Drawing for the job (mm, zero at the part's lowest x, y, z). A direction names the side the tool comes from. Give positions to 0.01 mm unless a question says otherwise; leave off trailing zeros. Write each loop counter-clockwise with the first axis right and the second up, starting at its lowest first coordinate (ties: lowest second). Pieces come first, ordered by that corner, then holes. Notation, with made-up numbers: (78, 20.5) - (96, 20.5) arc R20 cw to (96, 40.5) - close; hole circle Ø8 at (-3.5, 24.25). An arc over 180 degrees is marked (long way). Write item = value, one per line. Start each with the question number.
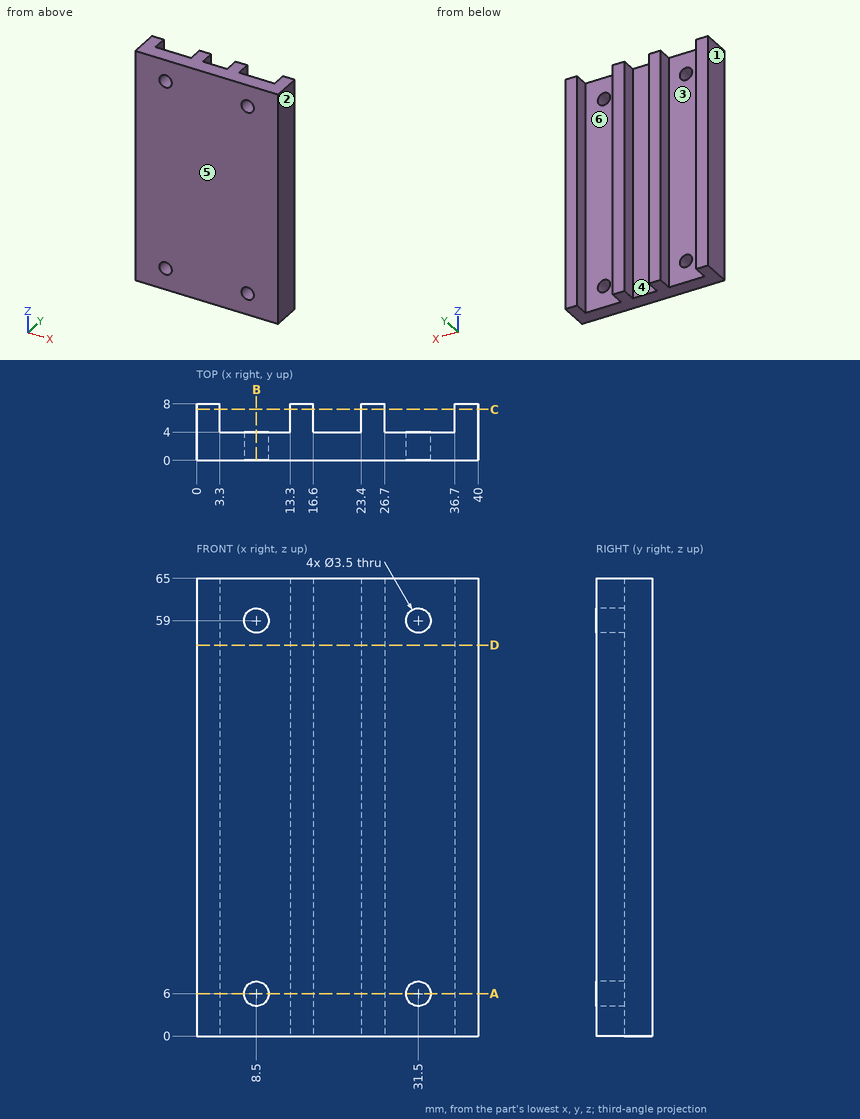
1. Pin check, flat tip, straight feed: pin 1 Ø3 at (x, z) = (6, 27) entering from +Y. Stop position of the tip, or through.
2. Wall check: line 1 along X through (y, z) = (4.25, 27); line 2 along Z through (x, y) = (31.5, 1.75); line 3 along X through (y, z) = (2.1, 6). Give the ranges that are in metal, low to high.
3. Cut at A-A (z = 6). Give the cut face in (x, y).
4. Cut at D-D (z = 55.5). Give the cut face in (x, y), then the cut area to 3 significant figures.
5. Cut at B-B (x = 8.5). Give the cut face in (y, z), then the cut area to 3 significant figures.
6. Cut at C-C (y = 7.25). Give the cut face in (x, z).
7. Mould opens along X. For the marked faces 1, 2, 3 and 4 say: +X half, -X half, draft (parallel to the pull), parting line (faces both ways), or undercut.
8. Tool access for the marked faces 5 and 6: list every direction of +Z, -Z, +X, -X, +Y, -Y with a clear straight run to the whole face (end or side of a thin tool).
Output:
q1.pin_1 = 4
q2.line_1 = 0 to 3.3, 13.3 to 16.6, 23.4 to 26.7, 36.7 to 40
q2.line_2 = 0 to 4.25, 7.75 to 57.25, 60.75 to 65
q2.line_3 = 0 to 6.75, 10.25 to 29.75, 33.25 to 40
q3.outline = (0, 0) - (6.75, 0) - (6.75, 4) - (3.3, 4) - (3.3, 8) - (0, 8) - close; (10.25, 0) - (29.75, 0) - (29.75, 4) - (26.7, 4) - (26.7, 8) - (23.4, 8) - (23.4, 4) - (16.6, 4) - (16.6, 8) - (13.3, 8) - (13.3, 4) - (10.25, 4) - close; (33.25, 0) - (40, 0) - (40, 8) - (36.7, 8) - (36.7, 4) - (33.25, 4) - close
q4.outline = (0, 0) - (40, 0) - (40, 8) - (36.7, 8) - (36.7, 4) - (26.7, 4) - (26.7, 8) - (23.4, 8) - (23.4, 4) - (16.6, 4) - (16.6, 8) - (13.3, 8) - (13.3, 4) - (3.3, 4) - (3.3, 8) - (0, 8) - close
q4.area = 213 mm2
q5.outline = (0, 0) - (4, 0) - (4, 4.25) - (0, 4.25) - close; (0, 7.75) - (4, 7.75) - (4, 57.25) - (0, 57.25) - close; (0, 60.75) - (4, 60.75) - (4, 65) - (0, 65) - close
q5.area = 232 mm2
q6.outline = (0, 0) - (3.3, 0) - (3.3, 65) - (0, 65) - close; (13.3, 0) - (16.6, 0) - (16.6, 65) - (13.3, 65) - close; (23.4, 0) - (26.7, 0) - (26.7, 65) - (23.4, 65) - close; (36.7, 0) - (40, 0) - (40, 65) - (36.7, 65) - close
q7.face_1 = -X half
q7.face_2 = +X half
q7.face_3 = undercut
q7.face_4 = undercut
q8.face_5 = +Z, -Z, +X, -X, -Y
q8.face_6 = +Z, -Z, +Y
